```python
from build123d import *

# Parameters (mm, degrees)
SKETCH_1_W      = 17.8
SKETCH_1_H      = 110.5
SKETCH_1_R      = 1.95
SKETCH_1_R_2    = 1.45
EXTRUDE_1_DEPTH = 3
FILLET_1_R      = 8


with BuildPart() as part:
    # 草图1 → 凸台-拉伸1 (new body)
    with BuildSketch(Plane.XY):
        with Locations((0, 47.25)):
            Rectangle(SKETCH_1_W, SKETCH_1_H)
        Circle(SKETCH_1_R, mode=Mode.SUBTRACT)
        with Locations((0, 57.5)):
            Circle(SKETCH_1_R_2, mode=Mode.SUBTRACT)
        with Locations((0, 97.5)):
            Circle(SKETCH_1_R_2, mode=Mode.SUBTRACT)
    extrude(amount=EXTRUDE_1_DEPTH)

    # 圆角1
    fillet_1_edges = [part.edges().sort_by_distance(p)[0] for p in [
        (8.9, -8, 1.5),
        (-8.9, -8, 1.5),
    ]]
    fillet(fillet_1_edges, radius=FILLET_1_R)


solid = part.part
```
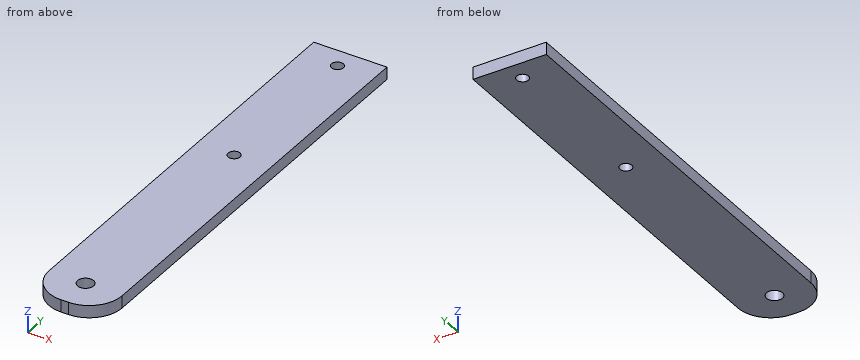
Check sheet for the modelled part. Datum: model origin and axes. Units: mm. Coordinates: 2 decimals unless noted, no trailing zeros. Write each loop counter-clockwise with the first axis right and the second up, starting at its lowest first coordinate (ties: lowest second). Pieces come first, ordered by that corner, then holes. Notation, with made-up numbers: (-10.5, 76.5) -> (10.5, 76.5) arc R15 ccw to (10.5, 90.5) -> close; hole circle Ø8 at (-11.75, 73.5). An arc over 180 degrees is marked (long way). Use a Markdown table: item, result.
1. Scan lines: line 1 along Y through (x, z) = (0, 1.75); line 2 along Y through (x, z) = (4.25, 1); line 3 along Y through (x, z) = (5.75, 0.6). Record each from-to range of solid material in increasing order.
Reported:
| item | result |
|---|---|
| line 1 | y = -8 to -1.95, 1.95 to 56.05, 58.95 to 96.05, 98.95 to 102.5 |
| line 2 | y = -7.26 to 102.5 |
| line 3 | y = -6.36 to 102.5 |
2. Sectioned sample at A-A (z = 1.6). Enter the section's corners in (x, y), plus the area to 3 significant figures.
Reported:
| item | result |
|---|---|
| outline | (-8.9, 0) arc R8 ccw to (-0.9, -8) -> (0.9, -8) arc R8 ccw to (8.9, 0) -> (8.9, 102.5) -> (-8.9, 102.5) -> close; hole circle Ø3.9 at (0, 0); hole circle Ø2.9 at (0, 57.5); hole circle Ø2.9 at (0, 97.5) |
| area | 1,910 mm2 |
3. Sectioned sample at B-B (y = 57.5). Enter the section's corners in (x, z).
Reported:
| item | result |
|---|---|
| outline | (-8.9, 0) -> (-1.45, 0) -> (-1.45, 3) -> (-8.9, 3) -> close; (1.45, 0) -> (8.9, 0) -> (8.9, 3) -> (1.45, 3) -> close |
4. Sectioned sample at C-C (x = -8). Enter the section's corners in (y, z).
Reported:
| item | result |
|---|---|
| outline | (-3.69, 0) -> (102.5, 0) -> (102.5, 3) -> (-3.69, 3) -> close |
